```python
from build123d import *

# Parameters (mm, degrees)
SKETCH1_R           = 9.525
SKETCH1_R_2         = 30.1625
BOSS_EXTRUDE1_DEPTH = 12.7


with BuildPart() as part:
    # Sketch1 → Boss-Extrude1 (new, symmetric)
    with BuildSketch(Plane(origin=(0, 0, 0), x_dir=(1, 0, 0), z_dir=(0, 1, 0))):
        with BuildLine():
            Line((-15.533043632, 38.240687501), (-72.019726416, 15.296275))
            ThreePointArc((-72.019726416, 15.296275), (-82.316508964, 0), (-72.019726416, -15.296275))
            Line((-72.019726416, -15.296275), (-15.533043632, -38.240687501))
            ThreePointArc((-15.533043632, -38.240687501), (-0.059033228, -41.274957784), (15.423593341, -38.28496302))
            Line((15.423593341, -38.28496302), (72.442928372, -15.313985208))
            ThreePointArc((72.442928372, -15.313985208), (82.737758003, -1.228011915), (74.64645973, 14.229318158))
            Line((74.64645973, 14.229318158), (70.194684869, 16.037591432))
            Line((70.194684869, 16.037591432), (15.533043632, 38.240687501))
            ThreePointArc((15.533043632, 38.240687501), (0, 41.275), (-15.533043632, 38.240687501))
        make_face()
        with Locations(Location((-65.806508964, 0, 0), (0, 0, 270))):
            Circle(SKETCH1_R, mode=Mode.SUBTRACT)
        with Locations(Location((0, 0, 0), (0, 0, 270))):
            Circle(SKETCH1_R_2, mode=Mode.SUBTRACT)
        with Locations(Location((66.273491036, 0, 0), (0, 0, 270))):
            Circle(SKETCH1_R, mode=Mode.SUBTRACT)
    extrude(amount=BOSS_EXTRUDE1_DEPTH, both=True)


solid = part.part
```
The model under review builds one solid part; all positions refer to its coordinate system, in mm. Round coordinates to 2 decimals unless told otherwise and drop trailing zeros. Loops run counter-clockwise (first coordinate to the right, second up) from the corner with the lowest first, then second, coordinate; pieces in that order, holes last. Notation, with made-up numbers: (70, -30) -> (90, -30) arc R13 ccw to (90, -7) -> close; hole circle Ø1 at (17, -19.75). An arc over 180 degrees is marked (long way). Answer in a Markdown table with one row per item.
1) Consider section D-D, the plane y = -0.5. Count the separate pieces of the cut face and the enclosed holes in it, plus the area to 3 significant figures.
Taken from the geometry:
| item | result |
|---|---|
| separate pieces | 1 |
| enclosed holes | 3 |
| area | 5,600 mm² |
2) Wall thickness on line 1 along X through (y, z) = (-1, 0); line 2 along Z through (x, y) = (-14.5, 2); line 3 along X through (y, z) = (0.75, 13.5): over which ranges is each line inside the solid? List them lowest first.
Taken from the geometry:
| item | result |
|---|---|
| line 1 | x = -82.32 to -75.33, -56.28 to -30.16, 30.16 to 56.75, 75.8 to 82.78 |
| line 2 | z = -38.64 to -26.45, 26.45 to 38.64 |
| line 3 | x = -75.31 to -26.97, 26.97 to 75.78 |
3) Draft analysis for pull direction X (two halves, no side actions). For faces 1 (the cylindrical face through (-82.314, 0.178, -0.274)), 2 (the cylindrical face through (-75.105, -0.178, -2.065)), 3 (the flat face through (43.53, 0.18, 26.96)), state which applies: pulls with the +X half, pulls with the -X half, needs draft (parallel to the pull), parting line crosses it, or undercut.
Taken from the geometry:
| item | result |
|---|---|
| face 1 | pulls with the -X half |
| face 2 | undercut |
| face 3 | pulls with the +X half |
4) Consider section C-C, the plane z = 17. Write out the cut boundary in (x, y).
Taken from the geometry:
| item | result |
|---|---|
| outline | (-67.83, -12.7) -> (-24.92, -12.7) -> (-24.92, 12.7) -> (-67.83, 12.7) -> close; (24.92, -12.7) -> (68.26, -12.7) -> (68.26, 12.7) -> (24.92, 12.7) -> close |
5) Consider section B-B, the plane z = 0. Write out the cut boundary in (x, y), plus the area to 3 significant figures.
Taken from the geometry:
| item | result |
|---|---|
| outline | (-82.32, -12.7) -> (-75.33, -12.7) -> (-75.33, 12.7) -> (-82.32, 12.7) -> close; (-56.28, -12.7) -> (-30.16, -12.7) -> (-30.16, 12.7) -> (-56.28, 12.7) -> close; (30.16, -12.7) -> (56.75, -12.7) -> (56.75, 12.7) -> (30.16, 12.7) -> close; (75.8, -12.7) -> (82.78, -12.7) -> (82.78, 12.7) -> (75.8, 12.7) -> close |
| area | 1,690 mm² |
6) For pin 1 Ø15 at (x, z) = (66.27, 0) entering from -Y; pin 2 Ø1 at (x, y) = (-4.5, 0) entering from -Z; pin 3 Ø3 at (x, y) = (43, -5.5) entering from -Z; pin 4 Ø1.5 at (x, y) = (48, -5.5) entering from +Z, all flat-tipped, find the tip position at first contact; note any pin that passes through.
Taken from the geometry:
| item | result |
|---|---|
| pin 1 | passes through |
| pin 2 | stops at z = -41.08 |
| pin 3 | stops at z = -27.69 |
| pin 4 | stops at z = 25.46 |
7) Consider section A-A, the plane x = 0. Write out the cut boundary in (y, z) (1 decimal).
Taken from the geometry:
| item | result |
|---|---|
| outline | (-12.7, -41.3) -> (12.7, -41.3) -> (12.7, -30.2) -> (-12.7, -30.2) -> close; (-12.7, 30.2) -> (12.7, 30.2) -> (12.7, 41.3) -> (-12.7, 41.3) -> close |
